from build123d import *

# Parameters (mm, degrees)
REDONDEO1_R          = 0.2
CHAFL_N1_SIZE        = 0.3
CHAFL_N2_SIZE        = 0.5
CORTAR_BARRER1_START = 3.956316317
CORTAR_BARRER1_DEPTH = 1.043683683


with BuildPart() as part:
    # Croquis1 → Revolución1 (revolve)
    with BuildSketch(Plane.XY):
        Polygon((0, 0), (0, -10), (2.5, -10), (2.5, 0), (4.25, 0), (4.25, 5), (0, 5), align=None)
    revolve(axis=Axis((0, -1001.198752701, 0), (0, 1, 0)))

    # Redondeo1
    redondeo1_edges = [part.edges().sort_by_distance(p)[0] for p in [
        (-2.5, 0, 0),
    ]]
    fillet(redondeo1_edges, radius=REDONDEO1_R)

    # Chaflán1
    chafl_n1_edges = [part.edges().sort_by_distance(p)[0] for p in [
        (-2.5, -10, 0),
    ]]
    chamfer(chafl_n1_edges, length=CHAFL_N1_SIZE)

    # Chaflán2
    chafl_n2_edges = [part.edges().sort_by_distance(p)[0] for p in [
        (-4.25, 5, 0),
        (-4.25, 0, 0),
    ]]
    chamfer(chafl_n2_edges, length=CHAFL_N2_SIZE)

    # Cortar-Barrer1: read off the stored shape, not the designer's step
    # Cortar-Barrer1 outline → Cortar-Barrer1 (cut)
    with BuildSketch(Plane(origin=(0, 0, 0), x_dir=(1, 0, 0), z_dir=(0, 1, 0)).offset(CORTAR_BARRER1_START)):
        Polygon((1.154700538, 2), (-1.154700538, 2), (-2.309401077, 0), (-1.154700538, -2), (1.154700538, -2), (2.309401077, 0), align=None)
    extrude(amount=CORTAR_BARRER1_DEPTH, mode=Mode.SUBTRACT)

    # Cortar-Barrer1 2: loft between two sections, ruled curve by curve
    cortar_barrer1_2_from = [
        Edge.make_line((-2.309401077, 3.956316317, 0), (-1.154700538, 3.956316317, -2)),
        Edge.make_line((-1.154700538, 3.956316317, 2), (-2.309401077, 3.956316317, 0)),
        Edge.make_line((-1.154700538, 3.956316317, -2), (1.154700538, 3.956316317, -2)),
        Edge.make_line((1.154700538, 3.956316317, 2), (-1.154700538, 3.956316317, 2)),
        Edge.make_line((1.154700538, 3.956316317, -2), (2.309401077, 3.956316317, 0)),
        Edge.make_line((2.309401077, 3.956316317, 0), (1.154700538, 3.956316317, 2)),
    ]
    cortar_barrer1_2_to = [
        Edge.make_line((-1.235376897, 3.257522104, 0), (-0.617688448, 3.257522104, -1.069867776)),
        Edge.make_line((-0.617688448, 3.257522104, 1.069867776), (-1.235376897, 3.257522104, 0)),
        Edge.make_line((-0.617688448, 3.257522104, -1.069867776), (0.617688448, 3.257522104, -1.069867776)),
        Edge.make_line((0.617688448, 3.257522104, 1.069867776), (-0.617688448, 3.257522104, 1.069867776)),
        Edge.make_line((0.617688448, 3.257522104, -1.069867776), (1.235376897, 3.257522104, 0)),
        Edge.make_line((1.235376897, 3.257522104, 0), (0.617688448, 3.257522104, 1.069867776)),
    ]
    cortar_barrer1_2 = Solid(Shell([*[Face.make_surface_from_curves(cortar_barrer1_2_from[k], cortar_barrer1_2_to[k]) for k in range(6)], Face(Wire(cortar_barrer1_2_from)), Face(Wire(cortar_barrer1_2_to))]))
    add(cortar_barrer1_2, mode=Mode.SUBTRACT)


solid = part.part
Geometry: final body of the model. Coordinates: model frame, mm. A direction names the side the tool comes from. Coordinates: 2 decimals unless noted, no trailing zeros. Write each loop counter-clockwise with the first axis right and the second up, starting at its lowest first coordinate (ties: lowest second). Pieces come first, ordered by that corner, then holes. Notation, with made-up numbers: (20.25, 22.25) - (41.25, 22.25) arc R25 ccw to (41.25, 50.25) - close; hole circle Ø5 at (20, 67.25). An arc over 180 degrees is marked (long way). Return JSON: item names as keys, results as strings.
Item 1: Pull-direction query (X, two-part tool) for faces 1 (the face through (-1.724, 4.471, -1.014)), 2 (the face through (1, 0, -3)), 3 (the face through (-0.54, -4.88, 2.44)), 4 (the face through (1.74, 4.47, -0.99)); classes: +X half, -X half, draft (parallel to the pull), parting line (faces both ways), or undercut.
Completed:
{"face 1": "undercut", "face 2": "draft", "face 3": "parting line", "face 4": "undercut"}
Item 2: Reachability of faces 5 (the face through (0, -10, 0)), 6 (the face through (-1.74, 4.47, 0.99)) from +Z, -Z, +X, -X, +Y, -Y: full face, straight path, thin tool, end or side. Return the list, or none.
Completed:
{"face 5": "+Z, -Z, +X, -X, -Y", "face 6": "+Y"}
Item 3: Section query A-A (y = -0.75). Output: boundary loops of the cut face in (x, z), and give its area (3 significant figures).
Completed:
{"outline": "circle Ø5 at (0, 0)", "area": "19.6 mm2"}
Item 4: Line query: L1, parallel to Y at x = 1.75, z = -2.5; L2, parallel to Y at x = 0.5, z = -0.75; L3, parallel to X at y = -5.75, z = -1.5. Output: solid intervals per line, ascending.
Completed:
{"L1": "y = 0 to 5", "L2": "y = -10 to 3.26", "L3": "x = -2 to 2"}
Item 5: Pin query (flat end, axial travel): pin 1 Ø1.1 at (x, z) = (0.5, -0.5) entering from +Y; pin 2 Ø2 at (x, z) = (-2.5, -3) entering from -Y; pin 3 Ø1 at (y, z) = (2, -1) entering from +X. Return the tip coordinate at first contact, or that it passes through.
Completed:
{"pin 1": "stops at y = 3.38", "pin 2": "stops at y = 0", "pin 3": "stops at x = 4.22"}
